from build123d import *

# Parameters (mm, degrees)
EXTRUDE_1_DEPTH     = 5
EXTRUDE_2_DEPTH     = 48
EXTRUDE_4_DEPTH     = 5
SKETCH_4_R          = 1.5
CUT_EXTRUDE_1_DEPTH = 4.5
SKETCH_5_R          = 11
EXTRUDE_5_DEPTH     = 2
SKETCH_6_R          = 4
CUT_EXTRUDE_2_DEPTH = 20


with BuildPart() as part:
    # 草图1 → 凸台-拉伸1 (new body)
    with BuildSketch(Plane.XY):
        with BuildLine():
            Line((-19.15, -21.15), (19.15, -21.15))
            ThreePointArc((19.15, -21.15), (20.564213562, -20.564213562), (21.15, -19.15))
            Line((21.15, -19.15), (21.15, 19.15))
            ThreePointArc((21.15, 19.15), (20.564213562, 20.564213562), (19.15, 21.15))
            Line((19.15, 21.15), (-19.15, 21.15))
            ThreePointArc((-19.15, 21.15), (-20.564213562, 20.564213562), (-21.15, 19.15))
            Line((-21.15, 19.15), (-21.15, -19.15))
            ThreePointArc((-21.15, -19.15), (-20.564213562, -20.564213562), (-19.15, -21.15))
        make_face()
    extrude(amount=EXTRUDE_1_DEPTH)

    # 草图2 → 凸台-拉伸2 (add)
    with BuildSketch(Plane.XY.offset(5)):
        with BuildLine():
            Line((-17.011566207, 15.988433793), (-15.988433793, 17.011566207))
            ThreePointArc((-15.988433793, 17.011566207), (-13.785943914, 18.483222894), (-11.187929962, 19))
            Line((-11.187929962, 19), (11.187929962, 19))
            ThreePointArc((11.187929962, 19), (13.785943914, 18.483222894), (15.988433793, 17.011566207))
            Line((15.988433793, 17.011566207), (17.011566207, 15.988433793))
            ThreePointArc((17.011566207, 15.988433793), (18.483222894, 13.785943914), (19, 11.187929962))
            Line((19, 11.187929962), (19, -11.187929962))
            ThreePointArc((19, -11.187929962), (18.483222894, -13.785943914), (17.011566207, -15.988433793))
            Line((17.011566207, -15.988433793), (15.988433793, -17.011566207))
            ThreePointArc((15.988433793, -17.011566207), (13.785943914, -18.483222894), (11.187929962, -19))
            Line((11.187929962, -19), (-11.187929962, -19))
            ThreePointArc((-11.187929962, -19), (-13.785943914, -18.483222894), (-15.988433793, -17.011566207))
            Line((-15.988433793, -17.011566207), (-17.011566207, -15.988433793))
            ThreePointArc((-17.011566207, -15.988433793), (-18.483222894, -13.785943914), (-19, -11.187929962))
            Line((-19, -11.187929962), (-19, 11.187929962))
            ThreePointArc((-19, 11.187929962), (-18.483222894, 13.785943914), (-17.011566207, 15.988433793))
        make_face()
    extrude(amount=EXTRUDE_2_DEPTH)

    # 草图3 → 凸台-拉伸4 (add)
    with BuildSketch(Plane.XY.offset(53)):
        with BuildLine():
            Line((-19.15, -21.15), (19.15, -21.15))
            ThreePointArc((19.15, -21.15), (20.564213562, -20.564213562), (21.15, -19.15))
            Line((21.15, -19.15), (21.15, 19.15))
            ThreePointArc((21.15, 19.15), (20.564213562, 20.564213562), (19.15, 21.15))
            Line((19.15, 21.15), (-19.15, 21.15))
            ThreePointArc((-19.15, 21.15), (-20.564213562, 20.564213562), (-21.15, 19.15))
            Line((-21.15, 19.15), (-21.15, -19.15))
            ThreePointArc((-21.15, -19.15), (-20.564213562, -20.564213562), (-19.15, -21.15))
        make_face()
    extrude(amount=EXTRUDE_4_DEPTH)

    # 草图4 → 切除-拉伸1 (cut)
    with BuildSketch(Plane.XY.offset(58)):
        with Locations((15.5, 15.5)):
            Circle(SKETCH_4_R)
        with Locations((15.5, -15.5)):
            Circle(SKETCH_4_R)
        with Locations((-15.5, -15.5)):
            Circle(SKETCH_4_R)
        with Locations((-15.5, 15.5)):
            Circle(SKETCH_4_R)
    extrude(amount=-CUT_EXTRUDE_1_DEPTH, mode=Mode.SUBTRACT)

    # 草图5 → 凸台-拉伸5 (add)
    with BuildSketch(Plane.XY.offset(58)):
        with Locations(Location((0, 0, 0), (0, 0, 180))):
            Circle(SKETCH_5_R)
    extrude(amount=EXTRUDE_5_DEPTH)

    # 草图6 → 切除-拉伸2 (cut)
    with BuildSketch(Plane.XY.offset(60)):
        Circle(SKETCH_6_R)
    extrude(amount=-CUT_EXTRUDE_2_DEPTH, mode=Mode.SUBTRACT)


solid = part.part
Verification items for the finished model (mm, model axes). A direction names the side the tool comes from. Coordinates: 2 decimals unless noted, no trailing zeros. Write each loop counter-clockwise with the first axis right and the second up, starting at its lowest first coordinate (ties: lowest second). Pieces come first, ordered by that corner, then holes. Notation, with made-up numbers: M 8,-7 L 12,-7 A31 ccw 12,22 Z; hole C 26,65.25 d2. An arc over 180 degrees is marked long. Use CSV: the item, a comma, the result in double quotes.
Q1. Section check B-B, the plane z = 35.5. Enter the section's corners in (x, y), and give its area (3 significant figures).
Computed values:
outline,"M -19,-11.19 A6.79 ccw -17.01,-15.99 L -15.99,-17.01 A6.79 ccw -11.19,-19 L 11.19,-19 A6.79 ccw 15.99,-17.01 L 17.01,-15.99 A6.79 ccw 19,-11.19 L 19,11.19 A6.79 ccw 17.01,15.99 L 15.99,17.01 A6.79 ccw 11.19,19 L -11.19,19 A6.79 ccw -15.99,17.01 L -17.01,15.99 A6.79 ccw -19,11.19 Z"
area,"1,390 mm²"
Q2. Mould release check, pull along Z, two halves, no side actions. Record for faces 6 (the flat face through (15, -15, 53.5)), 7 (the cylindrical face through (20.58, 20.55, 2.46)), 8 (the flat face through (0, 19, 29)): pulls with the +Z half, pulls with the -Z half, needs draft (parallel to the pull), parting line crosses it, or undercut.
Computed values:
face 6,"pulls with the +Z half"
face 7,"needs draft"
face 8,"undercut"
Q3. Section check C-C, the plane y = 0. Enter the section's corners in (x, z).
Computed values:
outline,"M -21.15,0 L 21.15,0 L 21.15,5 L 19,5 L 19,53 L 21.15,53 L 21.15,58 L 11,58 L 11,60 L 4,60 L 4,40 L -4,40 L -4,60 L -11,60 L -11,58 L -21.15,58 L -21.15,53 L -19,53 L -19,5 L -21.15,5 Z"
Q4. Go/stop test with flat-tipped pins: P1, Ø5, axis at y = 5.5, z = 35.5, coming from the -X side; P2, Ø2.5, axis at x = 0, y = 1.5, coming from the +Z side; P3, Ø1.5, axis at x = 16, y = -15.5, coming from the +Z side. Record where each tip stops, or that it passes through.
Computed values:
P1,"x = -19"
P2,"z = 40"
P3,"z = 53.5"
Q5. Section check A-A, the plane z = 42.5. Enter the section's corners in (x, y).
Computed values:
outline,"M -19,-11.19 A6.79 ccw -17.01,-15.99 L -15.99,-17.01 A6.79 ccw -11.19,-19 L 11.19,-19 A6.79 ccw 15.99,-17.01 L 17.01,-15.99 A6.79 ccw 19,-11.19 L 19,11.19 A6.79 ccw 17.01,15.99 L 15.99,17.01 A6.79 ccw 11.19,19 L -11.19,19 A6.79 ccw -15.99,17.01 L -17.01,15.99 A6.79 ccw -19,11.19 Z; hole C 0,0 d8"
Q6. Thickness scan on line 1 along Y through (x, z) = (15.5, 55.85); line 2 along Y through (x, z) = (-15, 55); line 3 along Z through (x, y) = (17, 17). Record the ranges inside material, lowest first. Write a range as [from, to].
Computed values:
line 1,"[-21.15, -17], [-14, 14], [17, 21.15]"
line 2,"[-21.15, -16.91], [-14.09, 14.09], [16.91, 21.15]"
line 3,"[0, 5], [53, 58]"
Q7. Set-up check for faces 1 (the flat face through (-19, 0, 29)), 2 (the cylindrical face through (18.5, -13.75, 28.66)), 3 (the cylindrical face through (14, -15.43, 55.78)), 4 (the flat face through (-20, 2, 5)), 5 (the cylindrical face through (13.75, 18.5, 28.66)): record each of +Z, -Z, +X, -X, +Y, -Y from which the full face is reachable in a straight line by a thin tool's end or side.
Computed values:
face 1,"-X, +Y, -Y"
face 2,"+X, -Y"
face 3,"+Z"
face 4,"none"
face 5,"+X, +Y"
